Here's how the part is built. I have some questions about the finished solid (model axes, mm). Round coordinates to 2 decimals unless told otherwise and drop trailing zeros. Write each loop counter-clockwise with the first axis right and the second up, starting at its lowest first coordinate (ties: lowest second). Pieces come first, ordered by that corner, then holes. Notation, with made-up numbers: (54, 61.5) - (112, 61.5) arc R6 cw to (112, 65.5) - close; hole circle Ø9 at (84.25, -6). An arc over 180 degrees is marked (long way). One line per item, written item: value. Start each with the question number.
Item 1: Imagine slicing it at B-B, the plane z = 0.5. Please give me the cut outline in (x, y).
Item 2: Imagine slicing it at A-A, the plane x = -1.5. Please give me the cut outline in (y, z).
Item 3: Imagine slicing it at C-C, the plane y = -1.9. Please give me the cut outline in (x, z), then the cut area to 3 significant figures.
Item 4: For P1, Ø2, axis at x = 1.5, z = -1.5, coming from the +Y side, with a flat end and sliding along its axis, tell me the tip position at first contact or that it passes through.
Item 5: If I drill on line 1 (Y direction, x = 3.5, z = -4.25); line 2 (X direction, y = -1.85, z = 4.5); line 3 (X direction, y = -4.55, z = 4), over which ranges is the centre line in solid material (lowest first)?
```python
from build123d import *

# Parameters (mm, degrees)
SKETCH1_W           = 8
SKETCH1_H           = 10
BOSS_EXTRUDE1_DEPTH = 5
CUT_EXTRUDE1_REACH  = 12
SKETCH2_W           = 7
SKETCH2_H           = 0.5
CUT_EXTRUDE3_DEPTH  = 5


with BuildPart() as part:
    # Sketch1 → Boss-Extrude1 (new body)
    with BuildSketch(Plane(origin=(0, 0, 0), x_dir=(1, 0, 0), z_dir=(0, 1, 0))):
        Rectangle(SKETCH1_W, SKETCH1_H)
    extrude(amount=-BOSS_EXTRUDE1_DEPTH)

    # Sketch2 → Cut-Extrude1 (cut, up to next)
    with BuildSketch(Plane(origin=(0, 0, -5), x_dir=(-1, 0, 0), z_dir=(0, 0, -1)), mode=Mode.PRIVATE) as cut_extrude1_sk1:
        with Locations((-0.5, -1.85)):
            Rectangle(SKETCH2_W, SKETCH2_H)
    cut_extrude1_tool1 = extrude(cut_extrude1_sk1.sketch, amount=-CUT_EXTRUDE1_REACH, mode=Mode.PRIVATE) & part.part
    add(cut_extrude1_tool1.solids().sort_by_distance((0.5, -1.85, -5))[0], mode=Mode.SUBTRACT)
    # Sketch2 → Cut-Extrude1 (cut, up to next)
    with BuildSketch(Plane(origin=(0, 0, -5), x_dir=(-1, 0, 0), z_dir=(0, 0, -1)), mode=Mode.PRIVATE) as cut_extrude1_sk2:
        with Locations((-0.5, -3.15)):
            Rectangle(SKETCH2_W, SKETCH2_H)
    cut_extrude1_tool2 = extrude(cut_extrude1_sk2.sketch, amount=-CUT_EXTRUDE1_REACH, mode=Mode.PRIVATE) & part.part
    add(cut_extrude1_tool2.solids().sort_by_distance((0.5, -3.15, -5))[0], mode=Mode.SUBTRACT)

    # Sketch3 → Cut-Extrude3 (cut)
    with BuildSketch(Plane(origin=(0, 0, 0), x_dir=(1, 0, 0), z_dir=(0, 1, 0))):
        with BuildLine():
            Line((2.500033416, 5), (4, 5))
            Line((4, 5), (4, 3.510012302))
            ThreePointArc((4, 3.510012302), (3.557147777, 4.564194168), (2.500033416, 5))
        make_face()
        with BuildLine():
            Line((4, -3.510012302), (4, -5))
            Line((4, -5), (2.500033416, -5))
            ThreePointArc((2.500033416, -5), (3.557147777, -4.564194168), (4, -3.510012302))
        make_face()
    extrude(amount=-CUT_EXTRUDE3_DEPTH, mode=Mode.SUBTRACT)


solid = part.part
```
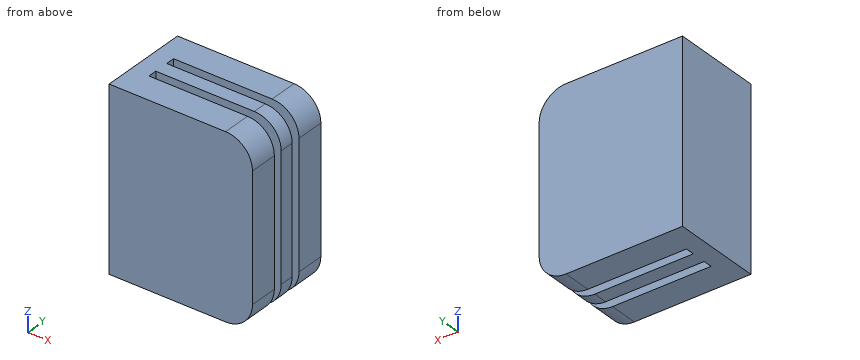
Values follow:
1. outline: (-4, -5) - (4, -5) - (4, -3.4) - (-3, -3.4) - (-3, -2.9) - (4, -2.9) - (4, -2.1) - (-3, -2.1) - (-3, -1.6) - (4, -1.6) - (4, 0) - (-4, 0) - close
2. outline: (-5, -5) - (-3.4, -5) - (-3.4, 5) - (-5, 5) - close; (-2.9, -5) - (-2.1, -5) - (-2.1, 5) - (-2.9, 5) - close; (-1.6, -5) - (0, -5) - (0, 5) - (-1.6, 5) - close
3. outline: (-4, -5) - (-3, -5) - (-3, 5) - (-4, 5) - close
3. area: 10.0 mm^2
4. P1: stops at y = 0
5. line 1: y = -5 to -3.4, -2.9 to -2.1, -1.6 to 0
5. line 2: x = -4 to -3
5. line 3: x = -4 to 3.91
